from build123d import *

# Parameters (mm, degrees)
F0_R      = 63.5
F1_DEPTH  = 12.7
F3_DEPTH  = 25.4
F6_DEPTH  = 12.7
F9_DEPTH  = 12.7
F10_R     = 9.525
F11_DEPTH = 88.901
F12_R     = 6.35
F13_DEPTH = 12.701
F14_R     = 3.81


with BuildPart() as f1:
    # F0 (on Top) → F1 (new body)
    with BuildSketch(Plane.XY):
        Circle(F0_R)
    extrude(amount=F1_DEPTH)

    # F2 (on Front) → F3 (join, symmetric)
    with BuildSketch(Plane.XZ):
        Polygon((-25.4, 50.8), (-25.4, 0), (0, 0), (0, 25.4), (-12.7, 25.4), (-12.7, 50.8), align=None)
        Polygon((0, 25.4), (0, 0), (25.4, 0), (25.4, 50.8), (12.7, 50.8), (12.7, 25.4), align=None)
    extrude(amount=F3_DEPTH, both=True)

    # F5 (on offset) → F6 (join)
    with BuildSketch(Plane.YZ.offset(25.4)):
        with BuildLine():
            Line((-25.4, 50.8), (25.4, 50.8))
            ThreePointArc((25.4, 50.8), (0, 76.2), (-25.4, 50.8))
        make_face()
    extrude(amount=-F6_DEPTH)

    # F8 (on offset) → F9 (join)
    with BuildSketch(Plane(origin=(-25.4, 0, 0), x_dir=(0, -1, 0), z_dir=(-1, 0, 0))):
        with BuildLine():
            Line((-25.4, 50.8), (25.4, 50.8))
            ThreePointArc((25.4, 50.8), (0, 76.2), (-25.4, 50.8))
        make_face()
    extrude(amount=-F9_DEPTH)

    # F10 (on face) → F11 (cut, through all)
    with BuildSketch(Plane.YZ.offset(25.4)):
        with Locations((0, 50.8)):
            Circle(F10_R)
    extrude(amount=-F11_DEPTH, mode=Mode.SUBTRACT)

    # F12 (on face) → F13 (cut, through all)
    with BuildSketch(Plane.XY.offset(12.7)):
        with Locations((0, 44.45)):
            Circle(F12_R)
        with Locations((44.45, 0)):
            Circle(F12_R)
        with Locations((0, -44.45)):
            Circle(F12_R)
        with Locations((-44.45, 0)):
            Circle(F12_R)
    extrude(amount=-F13_DEPTH, mode=Mode.SUBTRACT)

    # F14
    f14_edges = [f1.edges().sort_by_distance(p)[0] for p in [
        (-25.4, 0, 12.7),
        (0, -25.4, 12.7),
        (25.4, 0, 12.7),
        (0, 25.4, 12.7),
    ]]
    fillet(f14_edges, radius=F14_R)


solid = f1.part
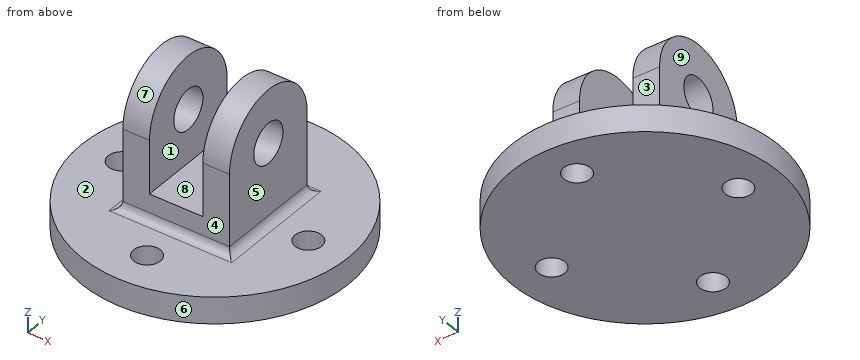
Geometry: final body of the model. Coordinates: model frame, mm. Face numbers are marked on the shaded views. A direction names the side the tool comes from. Round coordinates to 2 decimals unless told otherwise and drop trailing zeros. Loops run counter-clockwise (first coordinate to the right, second up) from the corner with the lowest first, then second, coordinate; pieces in that order, holes last. Notation, with made-up numbers: M 28,-10.5 L 64,-10.5 A24 ccw 64,11.5 Z; hole C 47,-14 d7. An arc over 180 degrees is marked long. One line per question, with ' | ' between items.
(1) Contact query for flat-ended pins moving along their axis: P1, Ø10.5, axis at x = 11.5, z = 42, coming from the -Y side; P2, Ø4, axis at y = 3.5, z = 38, coming from the -X side; P3, Ø8, axis at x = -12, y = -16.5, coming from the -Z side; P4, Ø7.5, axis at x = 5, y = 12.5, coming from the +Z side. Output: stop coordinate, or through.
Check result:
P1: stops at y = -25.4 | P2: stops at x = -25.4 | P3: stops at z = 0 | P4: stops at z = 25.4
(2) Cut plane B-B on y = 0. Give the number of separate pieces and of enclosed holes in the cut face, plus the area to 3 significant figures.
Check result:
separate pieces: 5 | enclosed holes: 0 | area: 2,750 mm2
(3) Cut plane A-A on z = 27.5. Return the cut outline in (x, y), plus the area to 3 significant figures.
Check result:
outline: M -25.4,-25.4 L -12.7,-25.4 L -12.7,25.4 L -25.4,25.4 Z; M 12.7,-25.4 L 25.4,-25.4 L 25.4,25.4 L 12.7,25.4 Z | area: 1,290 mm2
(4) Access query for the marked faces 1, 2, 3, 4 and 5. Directions: +Z, -Z, +X, -X, +Y, -Y. A direction counts if a zero-diameter tool reaches every point of the face in a straight line with its end or side. Return the directions, or none.
Check result:
face 1: +Z, +Y, -Y | face 2: +Z | face 3: +Z, +X, -X, +Y | face 4: +Z, +X, -X, -Y | face 5: +Z, +X, +Y, -Y
(5) Material intervals for line 1 along Y through (x, z) = (0, 8.25); line 2 along Z through (x, y) = (18, 0) (3 decimals); line 3 along Y through (x, z) = (46, 5.5) (3 decimals), sorted ascending. Write a range as from..to.
Check result:
line 1: y = -63.5..-50.8, -38.1..38.1, 50.8..63.5 | line 2: z = 0..41.275, 60.325..76.2 | line 3: y = -43.775..-6.158, 6.158..43.775
(6) Pull-direction query (X, two-part tool) for the marked faces 6, 7, 8 and 9; classes: +X half, -X half, draft (parallel to the pull), parting line (faces both ways), or undercut.
Check result:
face 6: parting line | face 7: draft | face 8: undercut | face 9: -X half
(7) Cut plane D-D on x = 0. Return the cut outline in (y, z).
Check result:
outline: M -63.5,0 L -50.8,0 L -50.8,12.7 L -63.5,12.7 Z; M -38.1,0 L 38.1,0 L 38.1,12.7 L 29.21,12.7 A3.81 cw 25.4,16.51 L 25.4,25.4 L -25.4,25.4 L -25.4,16.51 A3.81 cw -29.21,12.7 L -38.1,12.7 Z; M 50.8,0 L 63.5,0 L 63.5,12.7 L 50.8,12.7 Z
(8) Cut plane C-C on x = 44.45. Return the cut outline in (y, z).
Check result:
outline: M -45.35,0 L -6.35,0 L -6.35,12.7 L -45.35,12.7 Z; M 6.35,0 L 45.35,0 L 45.35,12.7 L 6.35,12.7 Z
